Geometry check sheet. Reference: the model listing, model coordinates, mm. Face numbers are marked on the shaded views. A direction names the side the tool comes from. Round coordinates to 2 decimals unless told otherwise and drop trailing zeros. Write each loop counter-clockwise with the first axis right and the second up, starting at its lowest first coordinate (ties: lowest second). Pieces come first, ordered by that corner, then holes. Notation, with made-up numbers: (21, -19) -> (77, -19) arc R20 ccw to (77, -1) -> close; hole circle Ø8 at (63.25, 35). An arc over 180 degrees is marked (long way). One line per question, with ' | ' between items.
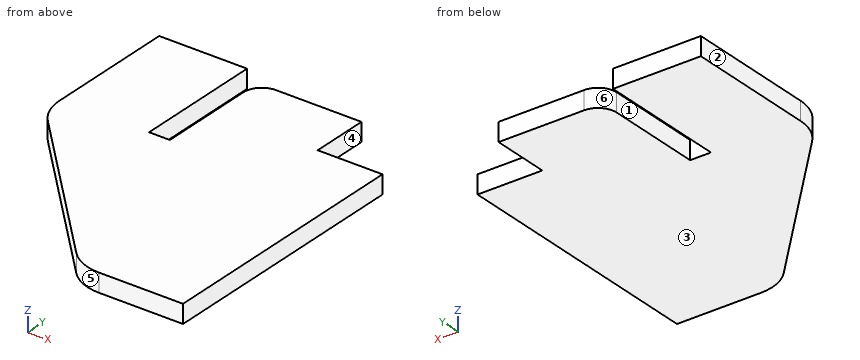
```python
from build123d import *

# Parameters (mm, degrees)
EXTRUDE_1_DEPTH = 8
FILLET_1_R      = 20


with BuildPart() as part:
    # 草图1 → 凸台-拉伸1 (new body)
    with BuildSketch(Plane.XY):
        with BuildLine():
            Line((0, 0), (0, 114))
            Line((0, 114), (-28, 114))
            Line((-28, 114), (-28, 139))
            Line((-28, 139), (-65, 139))
            ThreePointArc((-65, 139), (-70.656854249, 136.656854249), (-73, 131))
            Line((-73, 131), (-73, 89))
            Line((-73, 89), (-82, 89))
            Line((-82, 89), (-82, 145))
            Line((-82, 145), (-120, 145))
            Line((-120, 145), (-120, 80))
            Line((-120, 80), (-45, 0))
            Line((-45, 0), (0, 0))
        make_face()
    extrude(amount=EXTRUDE_1_DEPTH)

    # 圆角1
    fillet_1_edges = [part.edges().sort_by_distance(p)[0] for p in [
        (-45, 0, 4),
        (-120, 80, 4),
    ]]
    fillet(fillet_1_edges, radius=FILLET_1_R)


solid = part.part
```
(1) Sectioned sample at D-D on y = 72.5. Record the cut outline in (x, z).
Resolved:
outline: (-112.97, 0) -> (0, 0) -> (0, 8) -> (-112.97, 8) -> close
(2) Go/stop test with flat-tipped pins: pin 1 (2.5 mm diameter, centred on x = -12, z = 3.5, fed in from +Y); pin 2 (1 mm diameter, centred on x = -104.5, z = 3.5, fed in from -Y); pin 3 (1.5 mm diameter, centred on y = 16, z = 5.5, fed in from -X). Record where each tip stops, or that it passes through.
Resolved:
pin 1: stops at y = 114 | pin 2: stops at y = 62.93 | pin 3: stops at x = -60.7
(3) Sectioned sample at C-C on x = -95. Record the cut outline in (y, z).
Resolved:
outline: (53.33, 0) -> (145, 0) -> (145, 8) -> (53.33, 8) -> close
(4) Access from +Z, -Z, +X, -X, +Y, -Y to the whole of each face (thin tool, end or side, straight path). Record for the marked faces 4, 5 and 6.
Resolved:
face 4: +Z, -Z, +X, +Y | face 5: +Z, -Z, -X, -Y | face 6: +Z, -Z, +Y
(5) Sectioned sample at A-A on y = 126. Record the cut outline in (x, z), then the cut area to 3 significant figures.
Resolved:
outline: (-120, 0) -> (-82, 0) -> (-82, 8) -> (-120, 8) -> close; (-73, 0) -> (-28, 0) -> (-28, 8) -> (-73, 8) -> close | area: 664 mm2
(6) Sectioned sample at B-B on z = 2.75. Record the cut outline in (x, y).
Resolved:
outline: (-120, 87.91) arc R20 ccw to (-114.59, 74.23) -> (-50.93, 6.32) arc R20 ccw to (-36.34, 0) -> (0, 0) -> (0, 114) -> (-28, 114) -> (-28, 139) -> (-65, 139) arc R8 ccw to (-73, 131) -> (-73, 89) -> (-82, 89) -> (-82, 145) -> (-120, 145) -> close
(7) Material ranges on line 1 (X direction, y = 120, z = 7.75); line 2 (X direction, y = 137, z = 2); line 3 (Y direction, x = -7, z = 4.75), recorded low to high.
Resolved:
line 1: x = -120 to -82, -73 to -28 | line 2: x = -120 to -82, -70.29 to -28 | line 3: y = 0 to 114
(8) Draft check along X on the marked faces 1, 2 and 3. Enter one of: +X half, -X half, draft (parallel to the pull), parting line (faces both ways), or undercut.
Resolved:
face 1: undercut | face 2: -X half | face 3: draft
